Check sheet for the modelled part. Datum: model origin and axes. Units: mm. A direction names the side the tool comes from. Round coordinates to 2 decimals unless told otherwise and drop trailing zeros. Write each loop counter-clockwise with the first axis right and the second up, starting at its lowest first coordinate (ties: lowest second). Pieces come first, ordered by that corner, then holes. Notation, with made-up numbers: (67, 38) -> (79, 38) arc R35 ccw to (79, 74) -> close; hole circle Ø1 at (36.5, -20). An arc over 180 degrees is marked (long way). Answer as a JSON object with one key per item and string values. Group by question number.
```python
from build123d import *

# Parameters (mm, degrees)
F0_W     = 26.141723
F0_H     = 48.671415
F1_DEPTH = 7.857718
F2_T     = -2.5
F3_R     = 5


with BuildPart() as f1:
    # F0 (on Front) → F1 (new body)
    with BuildSketch(Plane.XZ):
        with Locations((0.317732, -7.252515)):
            Rectangle(F0_W, F0_H)
    extrude(amount=F1_DEPTH)

    # F2
    f2_openings = [f1.faces().sort_by_distance(p)[0] for p in [
        (0.317732, -7.857718, -7.252515),
    ]]
    offset(amount=F2_T, openings=f2_openings)

    # F3
    f3_edges = [f1.edges().sort_by_distance(p)[0] for p in [
        (13.388594, -3.928859, 17.083192),
        (-12.753129, -3.928859, 17.083192),
        (-12.753129, -3.928859, -31.588223),
        (13.388594, -3.928859, -31.588223),
    ]]
    fillet(f3_edges, radius=F3_R)


solid = f1.part
```
(1) Release check for a two-part mould opening along X. For faces 1 (the cylindrical face through (11.96, -3.98, 15.58)), 2 (the flat face through (-10.253, -5, -8)), 3 (the flat face through (0, -4, 17.083)), 4 (the flat face through (-12.753, -4, -8)) record: pulls with the +X half, pulls with the -X half, needs draft (parallel to the pull), parting line crosses it, or undercut.
(2) Section check C-C on z = -21. Record the cut outline in (x, y), then the cut area to 3 significant figures.
(3) Access from +Z, -Z, +X, -X, +Y, -Y to the whole of each face (thin tool, end or side, straight path). Record for faces 5 (the cylindrical face through (-11.327, -3.984, 15.58)), 6 (the flat face through (10.889, -5, -8)).
(4) Section check A-A on y = -5.75. Record the cut outline in (x, z).
(5) Go/stop test with flat-tipped pins: pin 1 Ø6.5 at (x, z) = (-4, -9) entering from -Y; pin 2 Ø2 at (x, z) = (-5, -9.5) entering from +Y. Record where each tip stops, or that it passes through.
(6) Scan lines: line 1 along Z through (x, y) = (6, -5); line 2 along X through (y, z) = (-3, -13); line 3 along Y through (x, z) = (-6.25, -10.5). Record each from-to range of solid material in increasing order.
(7) Section check B-B on x = -1. Record the cut outline in (y, z), then the cut area to 3 significant figures.
Data:
{
 "1": {"face 1": "pulls with the +X half", "face 2": "undercut", "face 3": "needs draft", "face 4": "pulls with the -X half"},
 "2": {"outline": "(-12.75, -7.86) -> (-10.25, -7.86) -> (-10.25, -2.5) -> (10.89, -2.5) -> (10.89, -7.86) -> (13.39, -7.86) -> (13.39, 0) -> (-12.75, 0) -> close", "area": "92.1 mm²"},
 "3": {"face 5": "+Z, -X, +Y, -Y", "face 6": "-Y"},
 "4": {"outline": "(-12.75, -26.59) arc R5 ccw to (-7.75, -31.59) -> (8.39, -31.59) arc R5 ccw to (13.39, -26.59) -> (13.39, 12.08) arc R5 ccw to (8.39, 17.08) -> (-7.75, 17.08) arc R5 ccw to (-12.75, 12.08) -> close; hole (-10.25, -29.09) -> (10.89, -29.09) -> (10.89, 14.58) -> (-10.25, 14.58) -> close"},
 "5": {"pin 1": "stops at y = -2.5", "pin 2": "stops at y = 0"},
 "6": {"line 1": "z = -31.59 to -29.09, 14.58 to 17.08", "line 2": "x = -12.75 to -10.25, 10.89 to 13.39", "line 3": "y = -2.5 to 0"},
 "7": {"outline": "(-7.86, -31.59) -> (0, -31.59) -> (0, 17.08) -> (-7.86, 17.08) -> (-7.86, 14.58) -> (-2.5, 14.58) -> (-2.5, -29.09) -> (-7.86, -29.09) -> close", "area": "148 mm²"}
}
